```python
from build123d import *

# Parameters (mm, degrees)
SKETCH1_R           = 19.05
BOSS_EXTRUDE2_DEPTH = 5.0038
SKETCH2_R           = 2.54
CUT_EXTRUDE1_DEPTH  = 7.5438
CIRPATTERN1_COUNT   = 5


with BuildPart() as part:
    # Sketch1 → Boss-Extrude2 (new body)
    with BuildSketch(Plane.XY):
        with BuildLine():
            Line((207.237556858, -115.975983371), (165.317532277, -85.519302738))
            Line((165.317532277, -85.519302738), (168.955516395, -80.512047172))
            ThreePointArc((168.955516395, -80.512047172), (150.561502758, -78.127913016), (132.170605091, -80.535965413))
            Line((132.170605091, -80.535965413), (135.828392716, -85.570478169))
            Line((135.828392716, -85.570478169), (93.908368135, -116.027158802))
            Line((93.908368135, -116.027158802), (90.270384017, -111.019903235))
            ThreePointArc((90.270384017, -111.019903235), (82.318874884, -127.776911795), (78.925968887, -146.011823976))
            Line((78.925968887, -146.011823976), (84.844393588, -144.08881122))
            Line((84.844393588, -144.08881122), (100.856418169, -193.368755668))
            Line((100.856418169, -193.368755668), (94.970036216, -195.281357105))
            ThreePointArc((94.970036216, -195.281357105), (108.449746946, -208.0218921), (124.743713387, -216.883635212))
            Line((124.743713387, -216.883635212), (124.743713387, -210.660635212))
            Line((124.743713387, -210.660635212), (176.559713387, -210.660635212))
            Line((176.559713387, -210.660635212), (176.559713387, -216.849943473))
            ThreePointArc((176.559713387, -216.849943473), (192.842141911, -207.967018576), (206.305272979, -195.208964837))
            Line((206.305272979, -195.208964837), (200.386848278, -193.285952081))
            Line((200.386848278, -193.285952081), (216.398872859, -144.006007633))
            Line((216.398872859, -144.006007633), (222.285254812, -145.918609069))
            ThreePointArc((222.285254812, -145.918609069), (218.868638328, -127.688124568), (210.895344483, -110.941470615))
            Line((210.895344483, -110.941470615), (207.237556858, -115.975983371))
        make_face()
        with Locations((150.608180965, -149.916372011)):
            Circle(SKETCH1_R, mode=Mode.SUBTRACT)
    extrude(amount=BOSS_EXTRUDE2_DEPTH)

    # Sketch2 → Cut-Extrude1 (cut)
    with BuildSketch(Plane(origin=(0, 0, 0), x_dir=(-1, 0, 0), z_dir=(0, 0, -1))):
        with Locations((-150.608395424, -86.435544776)):
            Circle(SKETCH2_R)
    cut_extrude1 = extrude(amount=-CUT_EXTRUDE1_DEPTH, mode=Mode.SUBTRACT)

    # CirPattern1: Cut-Extrude1 ×5 about axis
    cirpattern1_axis = Axis((150.608180965, -149.916372011, 0), (0, 0, 1))
    for i in range(1, CIRPATTERN1_COUNT):
        add(cut_extrude1.rotate(cirpattern1_axis, i * 360 / CIRPATTERN1_COUNT), mode=Mode.SUBTRACT)


solid = part.part
```
The model under review builds one solid part; all positions refer to its coordinate system, in mm. A direction names the side the tool comes from. Give positions to 0.01 mm unless a question says otherwise; leave off trailing zeros. Write each loop counter-clockwise with the first axis right and the second up, starting at its lowest first coordinate (ties: lowest second). Pieces come first, ordered by that corner, then holes. Notation, with made-up numbers: (-0.75, 87.25) -> (9.25, 87.25) arc R19 cw to (9.25, 112.25) -> close; hole circle Ø5 at (-19.75, -10.75). An arc over 180 degrees is marked (long way). Answer in a Markdown table with one row per item.
1) For L1, parallel to X at y = -202, z = 2.15 (3 decimals); L2, parallel to X at y = -140, z = 0.7; L3, parallel to X at y = -159.5, z = 1.4, list the stretches that pass through material, from the lowest coordinate up. Write a range as [from, to].
Worked answers:
| item | result |
|---|---|
| L1 | [101.203, 110.861], [115.729, 185.487], [190.355, 200.013] |
| L2 | [79.51, 134.34], [166.87, 221.71] |
| L3 | [89.85, 134.14], [167.07, 211.36] |
2) Add section C-C on y = -98. State the section outline as (x, z) points, plus the area to 3 significant figures.
Worked answers:
| item | result |
|---|---|
| outline | (118.72, 0) -> (182.5, 0) -> (182.5, 5) -> (118.72, 5) -> close |
| area | 319 mm² |
3) Add section D-D on x = 121.5. State the section outline as (y, z) points.
Worked answers:
| item | result |
|---|---|
| outline | (-215.54, 0) -> (-95.98, 0) -> (-95.98, 5) -> (-215.54, 5) -> close |
4) Tool access review of faces 5 (the flat face through (219.3, -144.95, 2.47)), 6 (the flat face through (97.954, -194.312, 2.467)), 7 (the cylindrical face through (208.477, -129.882, 2.467)), 8 (the flat face through (167.11, -83.05, 2.47)): name each direction out of +Z, -Z, +X, -X, +Y, -Y from which nothing blocks a thin tool from reaching the whole face with its end or side.
Worked answers:
| item | result |
|---|---|
| face 5 | +Z, -Z, -Y |
| face 6 | +Z, -Z, -X |
| face 7 | +Z, -Z |
| face 8 | +Z, -Z, +X |
5) Add section A-A on x = 144. State the section outline as (y, z) points.
Worked answers:
| item | result |
|---|---|
| outline | (-210.66, 0) -> (-167.78, 0) -> (-167.78, 5) -> (-210.66, 5) -> close; (-132.05, 0) -> (-78.43, 0) -> (-78.43, 5) -> (-132.05, 5) -> close |
6) Clearance check with flat-ended pins moving along their axes: P1, Ø2.5, axis at x = 157, z = 2.5, coming from the -Y side; P2, Ø2, axis at x = 135, z = 1, coming from the +Y side; P3, Ø1, axis at x = 120.5, z = 4, coming from the -Y side. State where each tip first meets the part, or that it passes through.
Worked answers:
| item | result |
|---|---|
| P1 | y = -210.66 |
| P2 | y = -79.63 |
| P3 | y = -215.31 |
7) Add section B-B on z = 3.35. State the section outline as (x, y) points.
Worked answers:
| item | result |
|---|---|
| outline | (78.93, -146.01) -> (84.84, -144.09) -> (100.86, -193.37) -> (94.97, -195.28) arc R71.79 ccw to (124.74, -216.88) -> (124.74, -210.66) -> (176.56, -210.66) -> (176.56, -216.85) arc R71.79 ccw to (206.31, -195.21) -> (200.39, -193.29) -> (216.4, -144.01) -> (222.29, -145.92) arc R71.79 ccw to (210.9, -110.94) -> (207.24, -115.98) -> (165.32, -85.52) -> (168.96, -80.51) arc R71.79 ccw to (132.17, -80.54) -> (135.83, -85.57) -> (93.91, -116.03) -> (90.27, -111.02) arc R71.79 ccw to start; hole circle Ø5.08 at (90.23, -130.3); hole circle Ø5.08 at (113.29, -201.27); hole circle Ø38.1 at (150.61, -149.92); hole circle Ø5.08 at (150.61, -86.44); hole circle Ø5.08 at (187.92, -201.27); hole circle Ø5.08 at (210.98, -130.3) |
8) Mouldability with a two-part tool opening along Y and no side actions: class faces 1 (the flat face through (81.844, -145.064, 2.467)), 2 (the flat face through (133.974, -83.018, 2.467)), 3 (the cylindrical face through (82.4, -127.53, 2.47)), 4 (the flat face through (124.744, -214, 2)) as +Y half, -Y half, draft (parallel to the pull), parting line (faces both ways), or undercut.
Worked answers:
| item | result |
|---|---|
| face 1 | -Y half |
| face 2 | undercut |
| face 3 | +Y half |
| face 4 | draft |
